Verification items for the finished model (mm, model axes). A direction names the side the tool comes from. Coordinates: 2 decimals unless noted, no trailing zeros. Write each loop counter-clockwise with the first axis right and the second up, starting at its lowest first coordinate (ties: lowest second). Pieces come first, ordered by that corner, then holes. Notation, with made-up numbers: (-8.75, 61) -> (45.25, 61) arc R20 ccw to (45.25, 98) -> close; hole circle Ø8 at (41, -15). An arc over 180 degrees is marked (long way). Use CSV: the item, a comma, the result in double quotes.
```python
from build123d import *

# Parameters (mm, degrees)
F0_W     = 50.8
F0_H     = 50.8
F0_W_2   = 25.4
F0_H_2   = 25.4
F1_DEPTH = 50.8
F3_DEPTH = 12.7
F5_DEPTH = 12.7
F7_DEPTH = 12.7
F9_DEPTH = 12.7


with BuildPart() as f1:
    # F0 (on Top) → F1 (new body)
    with BuildSketch(Plane.XY):
        with Locations((25.4, 25.4)):
            Rectangle(F0_W, F0_H)
        with Locations((25.4, 25.4)):
            Rectangle(F0_W_2, F0_H_2, mode=Mode.SUBTRACT)
    extrude(amount=F1_DEPTH)

    # F2 (on face) → F3 (cut)
    with BuildSketch(Plane.YZ.offset(50.8)):
        Polygon((12.7, 30.48), (12.7, 0), (38.1, 0), align=None)
        Polygon((38.1, 20.32), (38.1, 50.8), (12.7, 50.8), align=None)
    extrude(amount=-F3_DEPTH, mode=Mode.SUBTRACT)

    # F4 (on face) → F5 (cut)
    with BuildSketch(Plane.XZ):
        Polygon((12.7, 30.48), (12.7, 0), (38.1, 0), align=None)
        Polygon((38.1, 20.32), (38.1, 50.8), (12.7, 50.8), align=None)
    extrude(amount=-F5_DEPTH, mode=Mode.SUBTRACT)

    # F6 (on face) → F7 (cut)
    with BuildSketch(Plane(origin=(0, 0, 0), x_dir=(0, -1, 0), z_dir=(-1, 0, 0))):
        Polygon((-38.1, 30.48), (-38.1, 0), (-12.7, 0), align=None)
        Polygon((-12.7, 20.32), (-12.7, 50.8), (-38.1, 50.8), align=None)
    extrude(amount=-F7_DEPTH, mode=Mode.SUBTRACT)

    # F8 (on face) → F9 (cut)
    with BuildSketch(Plane(origin=(0, 50.8, 0), x_dir=(-1, 0, 0), z_dir=(0, 1, 0))):
        Polygon((-38.1, 30.48), (-38.1, 0), (-12.7, 0), align=None)
        Polygon((-12.7, 20.32), (-12.7, 50.8), (-38.1, 50.8), align=None)
    extrude(amount=-F9_DEPTH, mode=Mode.SUBTRACT)


solid = f1.part
```
1) Set-up check for faces 1 (the flat face through (25.2, 6.3, 35.8)), 2 (the flat face through (25, 38.1, 26)), 3 (the flat face through (6.3, 25.6, 35.8)), 4 (the flat face through (44.5, 25.2, 35.8)): record each of +Z, -Z, +X, -X, +Y, -Y from which the full face is reachable in a straight line by a thin tool's end or side.
Return value:
face 1,"+Z, -Y"
face 2,"none"
face 3,"+Z, -X"
face 4,"+Z, +X"
2) Cross-section at C-C (z = 32). Record the boundary of the cut face in (x, y), plus the area to 3 significant figures.
Return value:
outline,"(0, 0) -> (28.37, 0) -> (28.37, 12.7) -> (0, 12.7) -> close; (0, 22.43) -> (12.7, 22.43) -> (12.7, 50.8) -> (0, 50.8) -> close; (22.43, 38.1) -> (50.8, 38.1) -> (50.8, 50.8) -> (22.43, 50.8) -> close; (38.1, 0) -> (50.8, 0) -> (50.8, 28.37) -> (38.1, 28.37) -> close"
area,"1,440 mm2"
3) Cross-section at A-A (x = 19). Record the boundary of the cut face in (y, z).
Return value:
outline,"(0, 22.92) -> (12.7, 22.92) -> (12.7, 43.24) -> (0, 43.24) -> close; (38.1, 7.56) -> (50.8, 7.56) -> (50.8, 27.88) -> (38.1, 27.88) -> close"
4) Cross-section at D-D (x = 46). Record the boundary of the cut face in (y, z), plus the area to 3 significant figures.
Return value:
outline,"(0, 0) -> (12.7, 0) -> (12.7, 30.48) -> (38.1, 0) -> (50.8, 0) -> (50.8, 50.8) -> (38.1, 50.8) -> (38.1, 20.32) -> (12.7, 50.8) -> (0, 50.8) -> close"
area,"1,810 mm2"
5) Cross-section at B-B (y = 23.5). Record the boundary of the cut face in (x, z).
Return value:
outline,"(0, 12.96) -> (12.7, 12.96) -> (12.7, 33.28) -> (0, 33.28) -> close; (38.1, 17.52) -> (50.8, 17.52) -> (50.8, 37.84) -> (38.1, 37.84) -> close"
6) Gauge pin test, flat ends, axial feed: pin 1 (4 mm diameter, centred on y = 16, z = 8, fed in from -X); pin 2 (1 mm diameter, centred on x = 31.5, y = 9, fed in from +Z); pin 3 (8 mm diameter, centred on x = 30.5, y = 9, fed in from +Z). Record the tip position at first contact, or that the pin passes through.
Return value:
pin 1,"x = 0"
pin 2,"z = 28.84"
pin 3,"z = 34.24"
7) Mould release check, pull along Y, two halves, no side actions. Record for faces 5 (the flat face through (25, 12.7, 25)), 6 (the flat face through (25, 0, 25)), 7 (the flat face through (44, 45, 0)): released by +Y, released by -Y, zero draft, split by the parting line, or undercut.
Return value:
face 5,"undercut"
face 6,"released by -Y"
face 7,"zero draft"
8) Scan lines: L1, parallel to Y at x = 8.5, z = 22; L2, parallel to X at y = 12, z = 24; L3, parallel to Y at x = 8.5, z = 30. Record each from-to range of solid material in increasing order.
Return value:
L1,"0 to 12.7, 14.1 to 31.03, 38.1 to 50.8"
L2,"0 to 12.7, 18.1 to 35.03, 38.1 to 50.8"
L3,"0 to 12.7, 20.77 to 37.7, 38.1 to 50.8"
